Geometry: final body of the model. Coordinates: model frame, mm. A direction names the side the tool comes from. Give positions to 0.01 mm unless a question says otherwise; leave off trailing zeros. Loops run counter-clockwise (first coordinate to the right, second up) from the corner with the lowest first, then second, coordinate; pieces in that order, holes last. Notation, with made-up numbers: (37.25, 57) - (91.25, 57) arc R22 cw to (91.25, 66) - close; hole circle Ø5 at (14.25, 87.5). An arc over 180 degrees is marked (long way). Answer in a Markdown table with one row per item.
from build123d import *

# Parameters (mm, degrees)
EXTRUDE_1_DEPTH     = 15
SKETCH_3_3_W        = 35
SKETCH_3_3_H        = 25
EXTRUDE_2_DEPTH     = 15
CUT_EXTRUDE_1_DEPTH = 245
SKETCH_7_R          = 21
CUT_EXTRUDE_2_DEPTH = 15
SKETCH_8_R          = 5
CUT_EXTRUDE_4_DEPTH = 10
EXTRUDE_START       = 15
SKETCH_8_5_W        = 16
SKETCH_8_5_H        = 25
SKETCH_8_5_R        = 5
EXTRUDE_4_DEPTH     = 15
CHAMFER_1_SIZE      = 5
FILLET_1_R          = 5
CHAMFER_2_SIZE      = 5


with BuildPart() as part:
    # Эскиз3 → Бобышка-Вытянуть1 (new body)
    with BuildSketch(Plane(origin=(0, 0, 0), x_dir=(1, 0, 0), z_dir=(0, 1, 0))):
        Polygon((-32, -75), (-32, 75), (-32, 100), (32, 100), (32, -100), (-32, -100), align=None)
    extrude(amount=EXTRUDE_1_DEPTH)

    # Эскиз3<3> → Бобышка-Вытянуть2 (add)
    with BuildSketch(Plane(origin=(0, 0, 0), x_dir=(1, 0, 0), z_dir=(0, 1, 0))):
        with Locations((-49.5, 87.5)):
            Rectangle(SKETCH_3_3_W, SKETCH_3_3_H)
        with Locations((-49.5, -87.5)):
            Rectangle(SKETCH_3_3_W, SKETCH_3_3_H)
    extrude(amount=EXTRUDE_2_DEPTH)

    # Эскиз6 → Вырез-Вытянуть1 (cut)
    with BuildSketch(Plane.XY.offset(110)):
        Polygon((-67, 15), (-32, 15), (-67, -0.312590504), align=None)
    extrude(amount=-CUT_EXTRUDE_1_DEPTH, mode=Mode.SUBTRACT)

    # Эскиз7 → Вырез-Вытянуть2 (cut)
    with BuildSketch(Plane(origin=(0, 15, 0), x_dir=(1, 0, 0), z_dir=(0, 1, 0))):
        with Locations(Location((7, 75, 0), (0, 0, 270))):
            Circle(SKETCH_7_R)
        with Locations(Location((7, 25, 0), (0, 0, 270))):
            Circle(SKETCH_7_R)
        with Locations(Location((7, -25, 0), (0, 0, 270))):
            Circle(SKETCH_7_R)
        with Locations(Location((7, -75, 0), (0, 0, 270))):
            Circle(SKETCH_7_R)
    extrude(amount=-CUT_EXTRUDE_2_DEPTH, mode=Mode.SUBTRACT)

    # Эскиз8 → Вырез-Вытянуть4 (cut)
    with BuildSketch(Plane(origin=(0, 0, 0), x_dir=(-1, 0, 0), z_dir=(0, -1, 0))):
        with Locations(Location((23, 75, 0), (0, 0, 90))):
            Circle(SKETCH_8_R)
        with Locations(Location((23, -75, 0), (0, 0, 90))):
            Circle(SKETCH_8_R)
    extrude(amount=-CUT_EXTRUDE_4_DEPTH, mode=Mode.SUBTRACT)

    # Эскиз8<5> → Бобышка-Вытянуть4 (add)
    # profile 1 of 2: a face of its own
    with BuildSketch(Plane(origin=(0, 0, 0), x_dir=(-1, 0, 0), z_dir=(0, -1, 0)).offset(EXTRUDE_START)):
        with Locations((24, 75)):
            Rectangle(SKETCH_8_5_W, SKETCH_8_5_H)
        with Locations(Location((23, 75, 0), (0, 0, 90))):
            Circle(SKETCH_8_5_R, mode=Mode.SUBTRACT)
    # profile 2 of 2: a face of its own
    with BuildSketch(Plane(origin=(0, 0, 0), x_dir=(-1, 0, 0), z_dir=(0, -1, 0)).offset(EXTRUDE_START)):
        with Locations((24, -75)):
            Rectangle(SKETCH_8_5_W, SKETCH_8_5_H)
        with Locations(Location((23, -75, 0), (0, 0, 90))):
            Circle(SKETCH_8_5_R, mode=Mode.SUBTRACT)
    extrude(amount=-EXTRUDE_4_DEPTH)

    # Фаска1
    # the kernel refuses this chamfer: 5 mm, written as the material it takes off along each edge
    with BuildSketch(Plane(origin=(32, 0, -112.85841494), x_dir=(0.027495876610586317, 0.9996219169112968, 0), z_dir=(0, 0, 1))) as chamfer_1_piece_1:
        Polygon((CHAMFER_1_SIZE * 0.999621916911, CHAMFER_1_SIZE * 0.0274958766106), (-CHAMFER_1_SIZE * 0.0274958766106, CHAMFER_1_SIZE * 0.999621916911), (0, 0), align=None)
    extrude(amount=225.71682988, mode=Mode.SUBTRACT)

    # Скругление1
    fillet_1_edges = [part.edges().sort_by_distance(p)[0] for p in [
        (-32, 15, 0),
    ]]
    fillet(fillet_1_edges, radius=FILLET_1_R)

    # Фаска2
    # the kernel refuses this chamfer: 5 mm, written as the material it adds along each edge
    with BuildSketch(Plane(origin=(-16, 0, 87.5), x_dir=(0.9996219169112968, 0.027495876610586372, 0), z_dir=(0, 0, -1))) as chamfer_2_piece_1_section:
        Polygon((CHAMFER_2_SIZE * 0.999621916911, CHAMFER_2_SIZE * 0.0274958766106), (-CHAMFER_2_SIZE * 0.0274958766106, CHAMFER_2_SIZE * 0.999621916911), (0, 0), align=None)
    chamfer_2_piece_1 = extrude(amount=25, mode=Mode.PRIVATE)
    chamfer_2_piece_1 = chamfer_2_piece_1 - Plane(origin=(7, -1.841726954, 75), x_dir=(0, 0, 1), z_dir=(0, 1, 0)) * Cylinder(21, 70, mode=Mode.PRIVATE)
    add(chamfer_2_piece_1)
    with BuildSketch(Plane(origin=(-16, 0, -62.5), x_dir=(0.9996219169112968, 0.027495876610586372, 0), z_dir=(0, 0, -1))) as chamfer_2_piece_2_section:
        Polygon((CHAMFER_2_SIZE * 0.999621916911, CHAMFER_2_SIZE * 0.0274958766106), (-CHAMFER_2_SIZE * 0.0274958766106, CHAMFER_2_SIZE * 0.999621916911), (0, 0), align=None)
    chamfer_2_piece_2 = extrude(amount=25, mode=Mode.PRIVATE)
    chamfer_2_piece_2 = chamfer_2_piece_2 - Plane(origin=(7, -1.841726954, -75), x_dir=(0, 0, 1), z_dir=(0, 1, 0)) * Cylinder(21, 70, mode=Mode.PRIVATE)
    add(chamfer_2_piece_2)


solid = part.part
Q1. Cut plane B-B (y = -10.75). Output: boundary loops of the cut face in (x, z), and give its area (3 significant figures).
Check values:
| item | result |
|---|---|
| outline | (-32, -87.5) - (-16, -87.5) - (-16, -62.5) - (-32, -62.5) - close; (-32, 62.5) - (-16, 62.5) - (-16, 87.5) - (-32, 87.5) - close; hole circle Ø10 at (-23, -75); hole circle Ø10 at (-23, 75) |
| area | 643 mm² |
Q2. Cut plane A-A (z = 25). Output: boundary loops of the cut face in (x, y).
Check values:
| item | result |
|---|---|
| outline | (-32, 0) - (-14, 0) - (-14, 15) - (-27, 15) arc R5 ccw to (-32, 10) - close; (28, 1) - (32, 5) - (32, 15) - (28, 15) - close |
Q3. Cut plane C-C (x = 7). Output: boundary loops of the cut face in (y, z).
Check values:
| item | result |
|---|---|
| outline | (0, -100) - (15, -100) - (15, -96) - (0, -96) - close; (0, -54) - (15, -54) - (15, -46) - (0, -46) - close; (0, -4) - (15, -4) - (15, 4) - (0, 4) - close; (0, 46) - (15, 46) - (15, 54) - (0, 54) - close; (0, 96) - (15, 96) - (15, 100) - (0, 100) - close |
Q4. Cut plane D-D (x = -23). Output: boundary loops of the cut face in (y, z).
Check values:
| item | result |
|---|---|
| outline | (-15, -87.5) - (0, -87.5) - (0, -100) - (15, -100) - (15, 100) - (0, 100) - (0, 87.5) - (-15, 87.5) - (-15, 80) - (10, 80) - (10, 70) - (-15, 70) - (-15, 62.5) - (0, 62.5) - (0, -62.5) - (-15, -62.5) - (-15, -70) - (10, -70) - (10, -80) - (-15, -80) - close |
Q5. Draft query along Z for faces 6 (the cylindrical face through (-13.5, 7.96, -79.55)), 7 (the flat face through (-24, -8, 87.5)), 8 (the flat face through (-15, -4, 75)). Return one class per face: pulls with the +Z half, pulls with the -Z half, needs draft (parallel to the pull), parting line crosses it, or undercut.
Check values:
| item | result |
|---|---|
| face 6 | undercut |
| face 7 | pulls with the +Z half |
| face 8 | needs draft |
Q6. Material intervals for line 1 along Z through (x, y) = (7, 6.5); line 2 along Z through (x, y) = (-23.5, -8.5); line 3 along Z through (x, y) = (-42, 6.5), sorted ascending.
Check values:
| item | result |
|---|---|
| line 1 | -100 to -96, -54 to -46, -4 to 4, 46 to 54, 96 to 100 |
| line 2 | -87.5 to -79.97, -70.03 to -62.5, 62.5 to 70.03, 79.97 to 87.5 |
| line 3 | -100 to -75, 75 to 100 |
Q7. Reachability of faces 1 (the cylindrical face through (-1.04, 7.6, 44.4)), 2 (the flat face through (-7, 7, -100)), 3 (the cylindrical face through (-24.915, -2.675, -79.619)), 4 (the flat face through (-16, -10, -75)), 5 (the flat face through (-24, -8, -62.5)) from +Z, -Z, +X, -X, +Y, -Y: full face, straight path, thin tool, end or side. Return the list, or none.
Check values:
| item | result |
|---|---|
| face 1 | +Y, -Y |
| face 2 | -Z, +X, -X, +Y, -Y |
| face 3 | -Y |
| face 4 | +Z, -Z, +X, -Y |
| face 5 | +X, -X, -Y |
Q8. First-contact query: pin 1 (7.5 mm diameter, centred on x = -22.5, y = -10.5, fed in from +Z); pin 2 (12.5 mm diameter, centred on x = -9, z = 85, fed in from -Y); pin 3 (1 mm diameter, centred on x = -29, y = -9, fed in from -Z). Flat tips, straight axial feed; report the tip coordinate or a pass-through.
Check values:
| item | result |
|---|---|
| pin 1 | z = 87.5 |
| pin 2 | y = -4.25 |
| pin 3 | z = -87.5 |
